Autodesk Inventor part; units mm, degrees
ref_plane "YZ Plane" through (0, 0, 0) normal (1, 0, 0) x (0, 1, 0)
ref_plane "XZ Plane" through (0, 0, 0) normal (0, 1, 0) x (-1, 0, 0)
ref_plane "XY Plane" through (0, 0, 0) normal (0, 0, 1) x (1, 0, 0)
sketch "Sketch1" plane through (0, 0, 0) normal (0, 1, 0) x (-1, 0, 0)
  line L0 (-15.1, 10.95) -> (15.1, 10.95)
  line L1 (15.1, 10.95) -> (15.1, -10.95)
  line L2 (15.1, -10.95) -> (-15.1, -10.95)
  line L3 (-15.1, -10.95) -> (-15.1, 10.95)
  line L4 (-15.1, 10.95) -> (15.1, -10.95) construction
  line L5 (15.1, 10.95) -> (-15.1, -10.95) construction
  line L6 (-3.5, 6.45) -> (9.4, 6.45)
  line L7 (9.4, 6.45) -> (9.4, -6.45)
  line L8 (9.4, -6.45) -> (-3.5, -6.45)
  line L9 (-3.5, -6.45) -> (-3.5, 6.45)
  line L10 (-3.5, 6.45) -> (9.4, -6.45) construction
  line L11 (9.4, 6.45) -> (-3.5, -6.45) construction
  circle A0 centre (2.95, 0) radius 6.45
  point P0 (0, 0)
  dimension "d0" = 21.9
  dimension "d1" = 30.2
  dimension "d3" = 12.9
  dimension "d4" = 18.6
extrude "Extrusion1" add sketch "Sketch1" along normal blind 1.15 contours L0 L1 L2 L3 | L6 A0 L9 | L6 L7 A0 | A0 | A0 L8 L9 | L7 L8 A0
extrude "Extrusion2" add sketch "Sketch1" against normal blind 8 contours A0
sketch "Sketch2" plane through (0, -8, 0) normal (0, -1, 0) x (1, 0, 0)
  line L0 (3.5, -6.45) -> (3.5, 6.45)
  line L1 (3.5, 6.45) -> (-9.4, 6.45)
  line L2 (-9.4, 6.45) -> (-9.4, -6.45)
  line L3 (-9.4, -6.45) -> (3.5, -6.45)
  line L4 (3.5, 6.45) -> (-9.4, -6.45)
  line L5 (3.5, -6.45) -> (-9.4, 6.45)
  circle A0 centre (-2.95, 0) radius 5.7
  point P0 (0, 0)
  dimension "d9" = 11.4
extrude "Extrusion3" add sketch "Sketch2" along normal blind 4.2 contours A0 L4 L5 | L5 L4 A0 | L4 L5 A0 | A0 L5 L4
sketch "Sketch3" plane through (0, 0, 0) normal (0, -1, 0) x (1, 0, 0)
  line L0 (15.1, -10.95) -> (-15.1, -10.95)
  line L1 (15.1, 10.95) -> (15.1, -10.95)
  line L2 (-15.1, 10.95) -> (15.1, 10.95)
  line L3 (-15.1, -10.95) -> (-15.1, 10.95)
  line L4 (15.1, -5) -> (7.1, -5)
  line L5 (7.1, -5) -> (7.1, 5)
  line L6 (7.1, 5) -> (15.1, 5)
  line L7 (15.1, 5) -> (15.1, -5)
  line L8 (15.1, -5) -> (7.1, 5) construction
  line L9 (7.1, -5) -> (15.1, 5) construction
  line L10 (15.1, 10.95) -> (15.1, -10.95)
  point P0 (0, 0)
  point P1 (11.1, 0)
  point P2 (15.1, 0)
  dimension "d12" = 10
  dimension "d13" = 8
extrude "Extrusion4" add sketch "Sketch3" along normal blind 5.7 contours L4 L5 L6 L1
sketch "Sketch4" plane through (0, 0, 0) normal (0, -1, 0) x (1, 0, 0)
  line L0 (7.1, 5) -> (15.1, 5)
  line L1 (15.1, 10.95) -> (15.1, 5)
  line L2 (-15.1, 10.95) -> (15.1, 10.95)
  line L3 (-15.1, -10.95) -> (-15.1, 10.95)
  line L4 (15.1, -10.95) -> (-15.1, -10.95)
  line L5 (15.1, -5) -> (15.1, -10.95)
  line L6 (15.1, -5) -> (7.1, -5)
  line L7 (7.1, -5) -> (7.1, 5)
  circle A0 centre (-11.825, -7.675) radius 1.575
  circle A1 centre (-11.825, 7.675) radius 1.575
  line L8 (-10.25, -9.6033) -> (-10.25, -6.1)
  line L9 (-10.25, -6.1) -> (-13.9455, -6.1)
  point P0 (0, 0)
  dimension "d16" = 3.15
  dimension "d17" = 3.15
  dimension "d18" = 4.85
  dimension "d19" = 3.275
  dimension "d20" = 3.275
  dimension "d21" = 4.85
extrude "Extrusion5" cut sketch "Sketch4" against normal through all contours A0 | A1
fillet "Fillet1" radius 2.5 4 edges at (-15.1, 0.575, -10.95) (-15.1, 0.575, 10.95) (15.1, 0.575, -10.95) (15.1, 0.575, 10.95)
sketch "Sketch5" plane through (0, 0, 0) normal (0, -1, 0) x (1, 0, 0)
  circle A0 centre (-11.825, 7.675) radius 1.575
  circle A1 centre (-11.825, -7.675) radius 1.575
  arc A2 (15.1, 8.45) -> (12.6, 10.95) centre (12.6, 8.45) ccw
  line L0 (-12.6, 10.95) -> (12.6, 10.95)
  arc A3 (-12.6, 10.95) -> (-15.1, 8.45) centre (-12.6, 8.45) ccw
  line L1 (-15.1, -8.45) -> (-15.1, 8.45)
  arc A4 (-15.1, -8.45) -> (-12.6, -10.95) centre (-12.6, -8.45) ccw
  line L2 (12.6, -10.95) -> (-12.6, -10.95)
  arc A5 (12.6, -10.95) -> (15.1, -8.45) centre (12.6, -8.45) ccw
  line L3 (15.1, -5) -> (15.1, -8.45)
  line L4 (15.1, -5) -> (7.1, -5)
  line L5 (7.1, -5) -> (7.1, 5)
  line L6 (7.1, 5) -> (15.1, 5)
  line L7 (15.1, 8.45) -> (15.1, 5)
  line L8 (-15.1, -8.45) -> (-15.1, -10.95)
  line L9 (-15.1, -10.95) -> (-12.6, -10.95)
  line L10 (-14.9891, 11.1013) -> (15.1, 10.95) construction
  line L11 (15.1, 10.95) -> (14.9891, -11.1013) construction
  line L12 (14.9891, -11.1013) -> (-15.1, -10.95) construction
  line L13 (-15.1, -10.95) -> (-14.9891, 11.1013) construction
  line L14 (12.6, 10.95) -> (15.1, 10.95)
  line L15 (15.1, 10.95) -> (15.1, 8.45)
  point P0 (0, 0)
decal "Decal1"
decal "Decal2"
decal "Decal3"
decal "Decal4"
equation "\"d20\" = d19"
equation "\"d21\" = d18"
properties part number "DF Robot DFR0029-R"
Source: CAD feature listing. Evaluate the final solid. Frame: model axes, mm. A direction names the side the tool comes from. Coordinates: 2 decimals unless noted, no trailing zeros. Loops run counter-clockwise (first coordinate to the right, second up) from the corner with the lowest first, then second, coordinate; pieces in that order, holes last. Notation, with made-up numbers: M -10.5,32.5 L 22.5,32.5 A25 cw 22.5,48.5 Z; hole C -18,-13.5 d3. An arc over 180 degrees is marked long. Use a Markdown table: item, result. Add a question column.
Q1. Section query C-C, the plane z = 0. Return loops of the section in (x, y).
Q2. Section query A-A, the plane y = -2.5. Return loops of the section in (x, z).
Q3. Draft query along Z for faces 1 (the cylindrical face through (-14.348, 0.583, -10.237)), 2 (the flat face through (0.2, 0.6, 10.95)), 3 (the cylindrical face through (-10.37, 0.57, -8.28)), 4 (the flat face through (7.1, -3, 0)). Return one class per face: pulls with the +Z half, pulls with the -Z half, needs draft (parallel to the pull), parting line crosses it, or undercut.
Q4. Section query D-D, the plane y = -11. Return loops of the section in (x, z), and give its area (3 significant figures).
Q5. Material intervals for L1, parallel to Y at x = 9, z = 0; L2, parallel to Y at x = 7, z = -4.25; L3, parallel to X at y = -4.75, z = -3.5, sorted ascending.
Q6. First-contact query: pin 1 (8 mm diameter, centred on x = -5, z = 6, fed in from -Y); pin 2 (5 mm diameter, centred on y = -5, z = 4, fed in from -X); pin 3 (2 mm diameter, centred on y = -10, z = 5.5, fed in from -X); pin 4 (9 mm diameter, centred on x = 9.5, z = 0, fed in from -Y). Flat tips, straight axial feed; report the tip coordinate or a pass-through.
Q7. Section query B-B, the plane x = 8.5. Return loops of the section in (y, z).
Q8. Access query for faces 5 (the flat face through (11, -3, 5)), 6 (the flat face through (11, -3, -5)), 7 (the flat face through (11, -5.7, 0)), 8 (the cylindrical face through (-1.552, -3.944, -6.297)). Directions: +Z, -Z, +X, -X, +Y, -Y. A direction counts if a zero-diameter tool reaches every point of the face in a straight line with its end or side. Return the directions, or none.
Result:
| question | item | result |
|---|---|---|
| 1 | outline | M -15.1,0 L -9.4,0 L -9.4,-8 L -8.65,-8 L -8.65,-12.2 L 2.75,-12.2 L 2.75,-8 L 3.5,-8 L 3.5,0 L 7.1,0 L 7.1,-5.7 L 15.1,-5.7 L 15.1,1.15 L -15.1,1.15 Z |
| 2 | outline | C -2.95,0 d12.9; M 7.1,-5 L 15.1,-5 L 15.1,5 L 7.1,5 Z |
| 3 | face 1 | pulls with the -Z half |
| 3 | face 2 | pulls with the +Z half |
| 3 | face 3 | undercut |
| 3 | face 4 | needs draft |
| 4 | outline | C -2.95,0 d11.4 |
| 4 | area | 102 mm2 |
| 5 | L1 | y = -5.7 to 1.15 |
| 5 | L2 | y = 0 to 1.15 |
| 5 | L3 | x = -8.37 to 2.47, 7.1 to 15.1 |
| 6 | pin 1 | stops at y = -12.2 |
| 6 | pin 2 | stops at x = -9.22 |
| 6 | pin 3 | stops at x = -6.45 |
| 6 | pin 4 | stops at y = -5.7 |
| 7 | outline | M -5.7,-5 L 0,-5 L 0,-10.95 L 1.15,-10.95 L 1.15,10.95 L 0,10.95 L 0,5 L -5.7,5 Z |
| 8 | face 5 | +Z, +X, -Y |
| 8 | face 6 | -Z, +X, -Y |
| 8 | face 7 | +Z, -Z, +X, -Y |
| 8 | face 8 | -Y |
